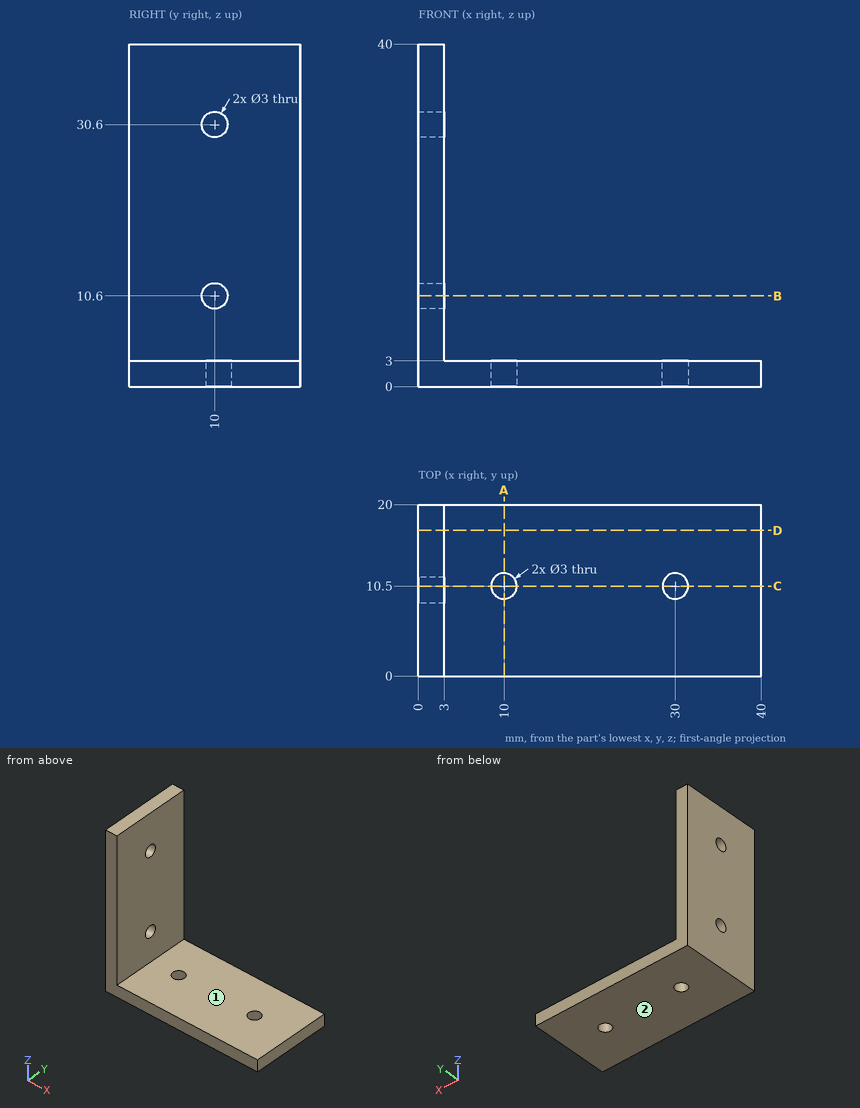
Geometry: see drawing. Coordinates: mm, zero at the bounding-box minimum. A direction names the side the tool comes from. Coordinates: 2 decimals unless noted, no trailing zeros. Loops run counter-clockwise (first coordinate to the right, second up) from the corner with the lowest first, then second, coordinate; pieces in that order, holes last. Notation, with made-up numbers: (-18.75, -37.75) - (-4.75, -37.75) arc R20 cw to (-4.75, -32.75) - close; hole circle Ø1 at (15.5, -22.5). An arc over 180 degrees is marked (long way). Return JSON: item names as keys, results as strings.
Q1. Section B-B, the plane z = 10.6. Return loops of the section in (x, y).
Results:
{"outline": "(0, 0) - (3, 0) - (3, 8.5) - (0, 8.5) - close; (0, 11.5) - (3, 11.5) - (3, 20) - (0, 20) - close"}
Q2. Access query for the marked faces 1 and 2. Directions: +Z, -Z, +X, -X, +Y, -Y. A direction counts if a zero-diameter tool reaches every point of the face in a straight line with its end or side. Return the directions, or none.
Results:
{"face 1": "+Z, +X, +Y, -Y", "face 2": "-Z, +X, -X, +Y, -Y"}
Q3. Section C-C, the plane y = 10.5. Return loops of the section in (x, z).
Results:
{"outline": "(0, 0) - (8.5, 0) - (8.5, 3) - (3, 3) - (3, 9.19) - (0, 9.19) - close; (0, 12.01) - (3, 12.01) - (3, 29.19) - (0, 29.19) - close; (0, 32.01) - (3, 32.01) - (3, 40) - (0, 40) - close; (11.5, 0) - (28.5, 0) - (28.5, 3) - (11.5, 3) - close; (31.5, 0) - (40, 0) - (40, 3) - (31.5, 3) - close"}
Q4. Contact query for flat-ended pins moving along their axis: P1, Ø10, axis at y = 12, z = 18, coming from the +X side; P2, Ø5, axis at x = 33, y = 11.5, coming from the +Z side; P3, Ø2.5, axis at y = 10, z = 30.6, coming from the +X side; P4, Ø6, axis at x = 12, z = 4, coming from the -Y side. Output: stop coordinate, or through.
Results:
{"P1": "x = 3", "P2": "z = 3", "P3": "through", "P4": "y = 0"}
Q5. Material intervals for line 1 along Y through (x, z) = (1.9, 30.6); line 2 along Y through (x, z) = (30, 1.75); line 3 along Z through (x, y) = (15.5, 3.25), sorted ascending.
Results:
{"line 1": "0 to 8.5, 11.5 to 20", "line 2": "0 to 9, 12 to 20", "line 3": "0 to 3"}
Q6. Section A-A, the plane x = 10. Return loops of the section in (y, z).
Results:
{"outline": "(0, 0) - (9, 0) - (9, 3) - (0, 3) - close; (12, 0) - (20, 0) - (20, 3) - (12, 3) - close"}
Q7. Section D-D, the plane y = 17. Return loops of the section in (x, z), plus the area to 3 significant figures.
Results:
{"outline": "(0, 0) - (40, 0) - (40, 3) - (3, 3) - (3, 40) - (0, 40) - close", "area": "231 mm2"}
